Check sheet for the modelled part. Datum: model origin and axes. Units: mm. A direction names the side the tool comes from. Round coordinates to 2 decimals unless told otherwise and drop trailing zeros. Write each loop counter-clockwise with the first axis right and the second up, starting at its lowest first coordinate (ties: lowest second). Pieces come first, ordered by that corner, then holes. Notation, with made-up numbers: (-18, 4.25) -> (26, 4.25) arc R34 cw to (26, 40.25) -> close; hole circle Ø10 at (-21, 52). An arc over 180 degrees is marked (long way). One line per item, written item: value.
from build123d import *

# Parameters (mm, degrees)
SKETCH_1_W          = 16
SKETCH_1_H          = 6
EXTRUDE_1_DEPTH     = 2
SKETCH_1_3_W        = 16
SKETCH_1_3_H        = 2
SKETCH_1_3_H_2      = 2.5
EXTRUDE_2_DEPTH     = 15
SKETCH_2_W          = 8
SKETCH_2_H          = 26
CUT_EXTRUDE_1_DEPTH = 2
EXTRUDE_3_DEPTH     = 2.5
EXTRUDE_4_DEPTH     = 5
EXTRUDE_5_DEPTH     = 1.5
CUT_EXTRUDE_START   = -6.633865
CUT_EXTRUDE_3_DEPTH = 6.633865
SKETCH_8_R          = 1.2
CUT_EXTRUDE_4_DEPTH = 8
SKETCH_9_W          = 1.2
SKETCH_9_H          = 1.320432063
EXTRUDE_6_DEPTH     = 2
EXTRUDE_7_DEPTH     = 12
SKETCH_10_W         = 2
SKETCH_10_H         = 8.943097661
EXTRUDE_8_DEPTH     = 10


with BuildPart() as part:
    # 草图1 → 凸台-拉伸1 (new body)
    with BuildSketch(Plane(origin=(0, 0, 0), x_dir=(1, 0, 0), z_dir=(0, 1, 0))):
        with Locations((0, 0.25)):
            Rectangle(SKETCH_1_W, SKETCH_1_H)
    extrude(amount=EXTRUDE_1_DEPTH)

    # 草图1<3> → 凸台-拉伸2 (add)
    with BuildSketch(Plane(origin=(0, 0, 0), x_dir=(1, 0, 0), z_dir=(0, 1, 0))):
        with Locations((0, 4.25)):
            Rectangle(SKETCH_1_3_W, SKETCH_1_3_H)
        with Locations((0, -4)):
            Rectangle(SKETCH_1_3_W, SKETCH_1_3_H_2)
    extrude(amount=EXTRUDE_2_DEPTH)

    # 草图2 → 切除-拉伸1 (cut)
    with BuildSketch(Plane(origin=(0, 0, -5.25), x_dir=(-1, 0, 0), z_dir=(0, 0, -1))):
        with Locations((0, 15)):
            Rectangle(SKETCH_2_W, SKETCH_2_H)
    extrude(amount=-CUT_EXTRUDE_1_DEPTH, mode=Mode.SUBTRACT)

    # 草图3 → 凸台-拉伸3 (add, symmetric)
    with BuildSketch(Plane(origin=(0, 0, 0), x_dir=(0, 0, -1), z_dir=(1, 0, 0))):
        Polygon((5.25, 0), (9.953715529, 0), (10.750589922, 15.09810313), (5.25, 15.388422994), align=None)
    extrude(amount=EXTRUDE_3_DEPTH, both=True)

    # 草图5 → 凸台-拉伸4 (add)
    with BuildSketch(Plane(origin=(2.5, 0, 0), x_dir=(0, 0, -1), z_dir=(1, 0, 0))):
        Polygon((5.25, 6.451105389), (3.822798244, 8.744995241), (3.822798244, 15.463750373), (5.25, 15.388422994), align=None)
    extrude(amount=-EXTRUDE_4_DEPTH)

    # 草图6 → 凸台-拉伸5 (add)
    with BuildSketch(Plane.ZY.offset(2.5)):
        Polygon((-5.25, 6.451105389), (-10.280190758, 6.185613084), (-10.750589922, 15.09810313), (-3.822798244, 15.463750373), (-3.822798244, 8.744995241), align=None)
    extrude_5 = extrude(amount=EXTRUDE_5_DEPTH)

    # 草图7 → 切除-拉伸3 (cut)
    with BuildSketch(Plane(origin=(0, -0.523895387, -9.926064452), x_dir=(-1, 0, 0), z_dir=(0, -0.052706408, -0.998610051)).offset(CUT_EXTRUDE_START)):
        Polygon((2.5, 6.718847324), (4, 9.892111055), (4, 6.718847324), align=None)
    cut_extrude_3 = extrude(amount=CUT_EXTRUDE_3_DEPTH, mode=Mode.SUBTRACT)

    # 镜向2: 凸台-拉伸5, 切除-拉伸3 across plane
    add(extrude_5.mirror(Plane(origin=(0, 0, 0), x_dir=(0, 0, 1), z_dir=(1, 0, 0))))
    add(cut_extrude_3.mirror(Plane(origin=(0, 0, 0), x_dir=(0, 0, 1), z_dir=(1, 0, 0))), mode=Mode.SUBTRACT)

    # 草图8 → 切除-拉伸4 (cut)
    with BuildSketch(Plane(origin=(4, 0, 0), x_dir=(0, 0, -1), z_dir=(1, 0, 0))):
        with Locations((8.533675648, 12.541707299)):
            Circle(SKETCH_8_R)
    extrude(amount=-CUT_EXTRUDE_4_DEPTH, mode=Mode.SUBTRACT)

    # 草图9 → 凸台-拉伸6 (add)
    with BuildSketch(Plane.XZ):
        with Locations((8.6, -2.910216032)):
            Rectangle(SKETCH_9_W, SKETCH_9_H)
        with Locations((-8.6, -2.910216032)):
            Rectangle(SKETCH_9_W, SKETCH_9_H)
    extrude(amount=-EXTRUDE_6_DEPTH)

    # 草图9<3> → 凸台-拉伸7 (add)
    with BuildSketch(Plane.XZ):
        Polygon((8, -3.570432063), (8, -5.25), (11.2, -5.25), (11.2, -2.25), (9.2, -2.25), (9.2, -3.570432063), align=None)
        Polygon((-8, -5.25), (-8, -3.570432063), (-9.2, -3.570432063), (-9.2, -2.25), (-11.2, -2.25), (-11.2, -5.25), align=None)
    extrude(amount=-EXTRUDE_7_DEPTH)

    # 草图10 → 凸台-拉伸8 (add)
    with BuildSketch(Plane.XY.offset(5.25)):
        with Locations((2.65, 4.471548831)):
            Rectangle(SKETCH_10_W, SKETCH_10_H)
        with Locations((-2.65, 4.471548831)):
            Rectangle(SKETCH_10_W, SKETCH_10_H)
    extrude(amount=EXTRUDE_8_DEPTH)


solid = part.part
Item 1: Tool access check on faces 1 (the flat face through (-8, 6, 3)), 2 (the flat face through (8, 6, 3)), 3 (the flat face through (8, 13, -4)). Record the directions out of +Z, -Z, +X, -X, +Y, -Y that give a thin tool (end or side, any length) a straight path to the whole face; none if there is none.
Result set:
face 1: +Z, -X, +Y, -Y
face 2: +Z, +X, +Y, -Y
face 3: +Z, +Y
Item 2: Depth check by flat-ended pin: pin 1 (7 mm diameter, centred on y = 3.5, z = 10.5, fed in from -X); pin 2 (2.5 mm diameter, centred on x = 10.5, y = 7, fed in from +Z); pin 3 (6.5 mm diameter, centred on y = 13, z = -7.5, fed in from +X); pin 4 (5 mm diameter, centred on y = 5, z = 8, fed in from +X). Enter the tip coordinate at first touch or a pass-through.
Result set:
pin 1: x = -3.65
pin 2: z = -2.25
pin 3: x = 11.2
pin 4: x = 3.65
Item 3: Sectioned sample at C-C (y = 4). State how many separate pieces and enclosed holes the cut face has, then the cut area to 3 significant figures.
Result set:
separate pieces: 4
enclosed holes: 0
area: 137 mm^2
Item 4: Material ranges on line 1 along Z through (x, y) = (5, 13.25); line 2 along X through (y, z) = (8, 10.5); line 3 along Z through (x, y) = (-1.75, 6.5), recorded low to high.
Result set:
line 1: -5.25 to -3.25, 2.75 to 5.25
line 2: -3.65 to -1.65, 1.65 to 3.65
line 3: -10.3 to -5.22, 2.75 to 15.25
Item 5: Sectioned sample at A-A (z = 8.75). Enter the section's corners in (x, y).
Result set:
outline: (-3.65, 0) -> (-1.65, 0) -> (-1.65, 8.94) -> (-3.65, 8.94) -> close; (1.65, 0) -> (3.65, 0) -> (3.65, 8.94) -> (1.65, 8.94) -> close
Item 6: Release check for a two-part mould opening along Z. For faces 4 (the flat face through (0, 12, -3.823)), 5 (the flat face through (-9, 7, -3.57)), 6 (the flat face through (-8, 13, -4)) record: pulls with the +Z half, pulls with the -Z half, needs draft (parallel to the pull), parting line crosses it, or undercut.
Result set:
face 4: undercut
face 5: pulls with the +Z half
face 6: needs draft
Item 7: Sectioned sample at B-B (x = 6.5). Enter the section's corners in (y, z).
Result set:
outline: (0, -5.25) -> (15, -5.25) -> (15, -3.25) -> (2, -3.25) -> (2, 2.75) -> (15, 2.75) -> (15, 5.25) -> (0, 5.25) -> close
Item 8: Sectioned sample at D-D (x = 1). Enter the section's corners in (y, z) (3 decimals), then the cut area to 3 significant figures.
Result set:
outline: (0, -9.954) -> (15.098, -10.751) -> (15.464, -3.823) -> (8.745, -3.823) -> (6.451, -5.25) -> (2, -5.25) -> (2, 2.75) -> (15, 2.75) -> (15, 5.25) -> (0, 5.25) -> close; hole circle Ø2.4 at (12.542, -8.534)
area: 138 mm^2
